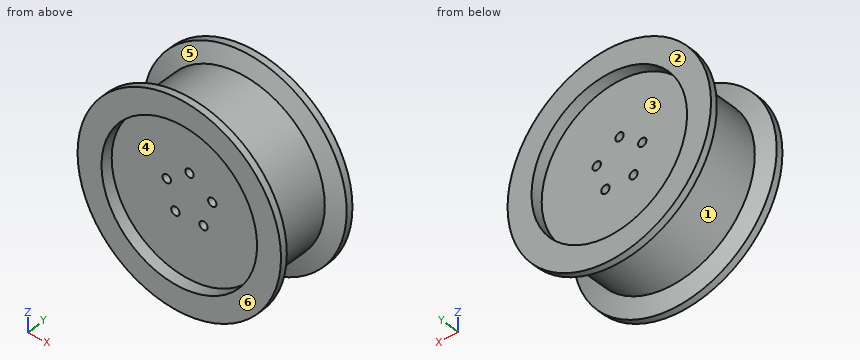
```python
from build123d import *

# Parameters (mm, degrees)
F0_R      = 215.9
F1_DEPTH  = 177.8
F5_R      = 165.1
F6_DEPTH  = 25.4
F7_R      = 165.1
F8_DEPTH  = 25.4
F9_R      = 8.89
F10_DEPTH = 152.401
F11_R     = 179.07
F11_R_2   = 177.8
F12_DEPTH = 158.75


with BuildPart() as f1:
    # F0 (on Front) → F1 (new body)
    with BuildSketch(Plane.XZ):
        Circle(F0_R)
    extrude(amount=-F1_DEPTH)

    # F2 (on Right) → F4 (revolve, cut)
    with BuildSketch(Plane.YZ):
        Polygon((165.534003, 222.889437), (88.9, 222.889437), (88.9, 161.774579), (92.761464, 161.774579), (146.810961, 161.774579), align=None)
        Polygon((88.9, 222.889437), (12.265997, 222.889437), (30.989039, 161.774579), (85.038536, 161.774579), (88.9, 161.774579), align=None)
    revolve(axis=Axis((0, 134.683609, 0), (0, 1, 0)), mode=Mode.SUBTRACT)

    # F5 (on face) → F6 (cut)
    with BuildSketch(Plane.XZ):
        Circle(F5_R)
    extrude(amount=-F6_DEPTH, mode=Mode.SUBTRACT)

    # F7 (on face) → F8 (cut)
    with BuildSketch(Plane(origin=(0, 177.8, 0), x_dir=(-1, 0, 0), z_dir=(0, 1, 0))):
        Circle(F7_R)
    extrude(amount=-F8_DEPTH, mode=Mode.SUBTRACT)

    # F9 (on face) → F10 (cut, through all)
    with BuildSketch(Plane.XZ.offset(-25.4)):
        with Locations((0, 50.8)):
            Circle(F9_R)
        with Locations((-48.313671, 15.698063)):
            Circle(F9_R)
        with Locations((-29.859491, -41.098063)):
            Circle(F9_R)
        with Locations((29.859491, -41.098063)):
            Circle(F9_R)
        with Locations((48.313671, 15.698063)):
            Circle(F9_R)
    extrude(amount=-F10_DEPTH, mode=Mode.SUBTRACT)

    # F11 (on face) → F12 (join)
    with BuildSketch(Plane(origin=(0, 177.8, 0), x_dir=(-1, 0, 0), z_dir=(0, 1, 0))):
        Circle(F11_R)
        Circle(F11_R_2, mode=Mode.SUBTRACT)
    extrude(amount=-F12_DEPTH)


solid = f1.part
```
Here's how the part is built. I have some questions about the finished solid (model axes, mm). Face numbers are marked on the shaded views. A direction names the side the tool comes from. Round coordinates to 2 decimals unless told otherwise and drop trailing zeros. Order: outer loops, then holes, each group sorted by start corner. A loop starts at its lowest first (then second) coordinate and runs counter-clockwise, first axis right, second up. Notation, with made-up numbers: (16.25, 19.5) -> (49.25, 19.5) arc R30 ccw to (49.25, 49.5) -> close; hole circle Ø10 at (36.5, 58.5). An arc over 180 degrees is marked (long way). Use a Markdown table: item, result. Add a question column.
(1) Suppose I cut it at B-B, the plane y = 57. Please give me the cut outline in (x, z), and give its area (3 significant figures).
(2) Suppose I cut it at C-C, the plane z = 0. Please give me the cut outline in (x, y).
(3) I need wall thicknesses on line 1 along X through (y, z) = (102, 1.5); line 2 along Z through (x, y) = (101.5, 32.5); line 3 along X through (y, z) = (125, 62). Which ranges of each line are inside material? Lowest first, please.
(4) For pin 1 Ø10 at (y, z) = (128, 40.5) entering from -X; pin 2 Ø5 at (x, z) = (-7.5, -91.5) entering from +Y; pin 3 Ø10 at (y, z) = (85, 8.5) entering from +X, each with a flat end and sliding along its axis, tell me the tip position at first contact or that it passes through.
(5) If we mould it in two halves opening along X, with no side actions, what happens to the marked faces 1, 2, 3 and 4? For each: released by +X, released by -X, zero draft, split by the parting line, or undercut.
(6) For the marked faces 5 and 6, which set-ups out of +Z, -Z, +X, -X, +Y, -Y let a thin tool reach every point of the face, with its end or its side?
(7) Suppose I cut it at A-A, the plane x = 0. Count the separate pieces of the cut face and the enclosed holes in it, and give its area (3 significant figures).
Verdict:
| question | item | result |
|---|---|---|
| 1 | outline | circle Ø358.14 at (0, 0); circle Ø323.55 at (0, 0); hole circle Ø355.6 at (0, 0); hole circle Ø17.78 at (-48.31, 15.7); hole circle Ø17.78 at (-29.86, -41.1); hole circle Ø17.78 at (0, 50.8); hole circle Ø17.78 at (29.86, -41.1); hole circle Ø17.78 at (48.31, 15.7) |
| 1 | area | 82,400 mm2 |
| 2 | outline | (-215.9, 0) -> (-165.1, 0) -> (-165.1, 25.4) -> (165.1, 25.4) -> (165.1, 0) -> (215.9, 0) -> (215.9, 14.41) -> (179.07, 25.69) -> (179.07, 152.11) -> (215.9, 163.39) -> (215.9, 177.8) -> (165.1, 177.8) -> (165.1, 152.4) -> (-165.1, 152.4) -> (-165.1, 177.8) -> (-215.9, 177.8) -> (-215.9, 163.39) -> (-179.07, 152.11) -> (-179.07, 25.69) -> (-215.9, 14.41) -> close; hole (-177.8, 26.08) -> (-161.77, 30.99) -> (-161.77, 146.81) -> (-177.8, 151.72) -> close; hole (161.77, 30.99) -> (177.8, 26.08) -> (177.8, 151.72) -> (161.77, 146.81) -> close |
| 3 | line 1 | -179.06 to -177.79, -161.77 to 161.77, 177.79 to 179.06 |
| 3 | line 2 | -147.53 to -145.98, -125.97 to 125.97, 145.98 to 147.53 |
| 3 | line 3 | -167.99 to -166.64, -149.42 to 149.42, 166.64 to 167.99 |
| 4 | pin 1 | x = -175.52 |
| 4 | pin 2 | y = 152.4 |
| 4 | pin 3 | x = 179.04 |
| 5 | face 1 | split by the parting line |
| 5 | face 2 | zero draft |
| 5 | face 3 | undercut |
| 5 | face 4 | undercut |
| 6 | face 5 | none |
| 6 | face 6 | +Z, -Z, +X, -X, -Y |
| 7 | separate pieces | 2 |
| 7 | enclosed holes | 2 |
| 7 | area | 43,700 mm2 |
